```python
from build123d import *

# Parameters (mm, degrees)
CROQUIS1_W                 = 42
CROQUIS1_H                 = 68
CROQUIS1_W_2               = 34
CROQUIS1_H_2               = 60
SALIENTE_EXTRUIR1_DEPTH    = 60
CROQUIS2_R                 = 1.5
CORTAR_EXTRUIR1_DEPTH      = 39
CORTAR_EXTRUIR1_DEPTH_BACK = 5
CROQUIS3_W                 = 42
CROQUIS3_H                 = 68
SALIENTE_EXTRUIR2_DEPTH    = 4
CROQUIS4_W                 = 64
CROQUIS4_H                 = 20
SALIENTE_EXTRUIR3_DEPTH    = 42
SALIENTE_EXTRUIR4_DEPTH    = 64
SALIENTE_EXTRUIR6_DEPTH    = 64
CROQUIS8_R                 = 50
SALIENTE_EXTRUIR7_DEPTH    = 350
SALIENTE_EXTRUIR8_START    = -4
SALIENTE_EXTRUIR8_DEPTH    = 64
CROQUIS11_R                = 1.5
CORTAR_EXTRUIR2_DEPTH      = 68
CORTAR_EXTRUIR2_DEPTH_BACK = 34
CROQUIS13_R                = 10
CROQUIS13_R_2              = 50
SALIENTE_EXTRUIR9_DEPTH    = 20


with BuildPart() as part:
    # Croquis1 → Saliente-Extruir1 (new body)
    with BuildSketch(Plane.XY):
        Rectangle(CROQUIS1_W, CROQUIS1_H)
        Rectangle(CROQUIS1_W_2, CROQUIS1_H_2, mode=Mode.SUBTRACT)
    extrude(amount=SALIENTE_EXTRUIR1_DEPTH)

    # Croquis2 → Cortar-Extruir1 (cut, two sides)
    with BuildSketch(Plane(origin=(-17, 0, 0), x_dir=(0, 0, -1), z_dir=(1, 0, 0))) as cortar_extruir1_sk:
        with Locations((-49.779, -10)):
            Circle(CROQUIS2_R)
        with Locations((-46.914797213, -3.085202787)):
            Circle(CROQUIS2_R)
        with Locations((-40, -0.221)):
            Circle(CROQUIS2_R)
        with Locations((-33.085202787, -3.085202787)):
            Circle(CROQUIS2_R)
        with Locations((-30.221, -10)):
            Circle(CROQUIS2_R)
        with Locations((-33.085202787, -16.914797213)):
            Circle(CROQUIS2_R)
        with Locations((-40, -19.779)):
            Circle(CROQUIS2_R)
        with Locations((-46.914797213, -16.914797213)):
            Circle(CROQUIS2_R)
    extrude(amount=CORTAR_EXTRUIR1_DEPTH, mode=Mode.SUBTRACT)
    extrude(cortar_extruir1_sk.sketch, amount=-CORTAR_EXTRUIR1_DEPTH_BACK, mode=Mode.SUBTRACT)

    # Croquis3 → Saliente-Extruir2 (add)
    with BuildSketch(Plane(origin=(0, 0, 0), x_dir=(-1, 0, 0), z_dir=(0, 0, -1))):
        Rectangle(CROQUIS3_W, CROQUIS3_H)
    extrude(amount=SALIENTE_EXTRUIR2_DEPTH)

    # Croquis4 → Saliente-Extruir3 (add)
    with BuildSketch(Plane(origin=(21, 0, 0), x_dir=(0, 0, -1), z_dir=(1, 0, 0))):
        with Locations((-28, -44)):
            Rectangle(CROQUIS4_W, CROQUIS4_H)
    extrude(amount=-SALIENTE_EXTRUIR3_DEPTH)

    # Croquis5 → Saliente-Extruir4 (add)
    with BuildSketch(Plane(origin=(0, 0, -4), x_dir=(-1, 0, 0), z_dir=(0, 0, -1))):
        with BuildLine():
            ThreePointArc((21, 34), (0, 38.754486973), (-21, 34))
            Line((-21, 34), (21, 34))
        make_face()
        with BuildLine():
            ThreePointArc((-21, -54), (0, -58.754486973), (21, -54))
            Line((21, -54), (-21, -54))
        make_face()
    extrude(amount=-SALIENTE_EXTRUIR4_DEPTH)

    # Croquis6 → Saliente-Extruir6 (add)
    with BuildSketch(Plane(origin=(0, 0, -4), x_dir=(-1, 0, 0), z_dir=(0, 0, -1))):
        with BuildLine():
            Line((-21, 34), (21, 34))
            Line((21, 34), (21, 35.376205218))
            ThreePointArc((21, 35.376205218), (0, 40), (-21, 35.376205218))
            Line((-21, 35.376205218), (-21, 34))
        make_face()
        with BuildLine():
            Line((-21, -55.376205218), (-21, -54))
            Line((-21, -54), (21, -54))
            Line((21, -54), (21, -55.376205218))
            ThreePointArc((21, -55.376205218), (0, -60), (-21, -55.376205218))
        make_face()
    extrude(amount=-SALIENTE_EXTRUIR6_DEPTH)

    # Croquis8 → Saliente-Extruir7 (add)
    with BuildSketch(Plane(origin=(0, 0, -4), x_dir=(-1, 0, 0), z_dir=(0, 0, -1))):
        with Locations((0, -10)):
            Circle(CROQUIS8_R)
    extrude(amount=SALIENTE_EXTRUIR7_DEPTH)

    # Croquis10 → Saliente-Extruir8 (add)
    with BuildSketch(Plane.XY.offset(SALIENTE_EXTRUIR8_START)):
        with BuildLine():
            Line((-21, 35.376205218), (-21, -55.376205218))
            ThreePointArc((-21, -55.376205218), (-24.056410521, -53.832512053), (-27, -52.083250825))
            Line((-27, -52.083250825), (-27, 32.083250825))
            ThreePointArc((-27, 32.083250825), (-24.056410521, 33.832512053), (-21, 35.376205218))
        make_face()
        with BuildLine():
            Line((21, 35.376205218), (21, -55.376205218))
            ThreePointArc((21, -55.376205218), (24.056410521, -53.832512053), (27, -52.083250825))
            Line((27, -52.083250825), (27, 32.083250825))
            ThreePointArc((27, 32.083250825), (24.056410521, 33.832512053), (21, 35.376205218))
        make_face()
    extrude(amount=SALIENTE_EXTRUIR8_DEPTH)

    # Croquis11 → Cortar-Extruir2 (cut, two sides)
    with BuildSketch(Plane(origin=(-17, 0, 0), x_dir=(0, 0, -1), z_dir=(1, 0, 0))) as cortar_extruir2_sk:
        with Locations((-49.779, -10)):
            Circle(CROQUIS11_R)
        with Locations((-46.914797213, -3.085202787)):
            Circle(CROQUIS11_R)
        with Locations((-40, -0.221)):
            Circle(CROQUIS11_R)
        with Locations((-33.085202787, -3.085202787)):
            Circle(CROQUIS11_R)
        with Locations((-30.221, -10)):
            Circle(CROQUIS11_R)
        with Locations((-33.085202787, -16.914797213)):
            Circle(CROQUIS11_R)
        with Locations((-40, -19.779)):
            Circle(CROQUIS11_R)
        with Locations((-46.914797213, -16.914797213)):
            Circle(CROQUIS11_R)
    extrude(amount=CORTAR_EXTRUIR2_DEPTH, mode=Mode.SUBTRACT)
    extrude(cortar_extruir2_sk.sketch, amount=-CORTAR_EXTRUIR2_DEPTH_BACK, mode=Mode.SUBTRACT)

    # Croquis13 → Saliente-Extruir9 (add)
    with BuildSketch(Plane(origin=(0, 0, -354), x_dir=(-1, 0, 0), z_dir=(0, 0, -1))):
        with BuildLine():
            Line((-50, -80), (50, -80))
            ThreePointArc((50, -80), (64.142135624, -74.142135624), (70, -60))
            Line((70, -60), (70, 40))
            ThreePointArc((70, 40), (64.142135624, 54.142135624), (50, 60))
            Line((50, 60), (-50, 60))
            ThreePointArc((-50, 60), (-64.142135624, 54.142135624), (-70, 40))
            Line((-70, 40), (-70, -60))
            ThreePointArc((-70, -60), (-64.142135624, -74.142135624), (-50, -80))
        make_face()
        with Locations((-50, 40)):
            Circle(CROQUIS13_R, mode=Mode.SUBTRACT)
        with Locations((-50, -60)):
            Circle(CROQUIS13_R, mode=Mode.SUBTRACT)
        with Locations((50, 40)):
            Circle(CROQUIS13_R, mode=Mode.SUBTRACT)
        with Locations((50, -60)):
            Circle(CROQUIS13_R, mode=Mode.SUBTRACT)
        with Locations((0, -10)):
            Circle(CROQUIS13_R_2, mode=Mode.SUBTRACT)
    extrude(amount=-SALIENTE_EXTRUIR9_DEPTH)


solid = part.part
```
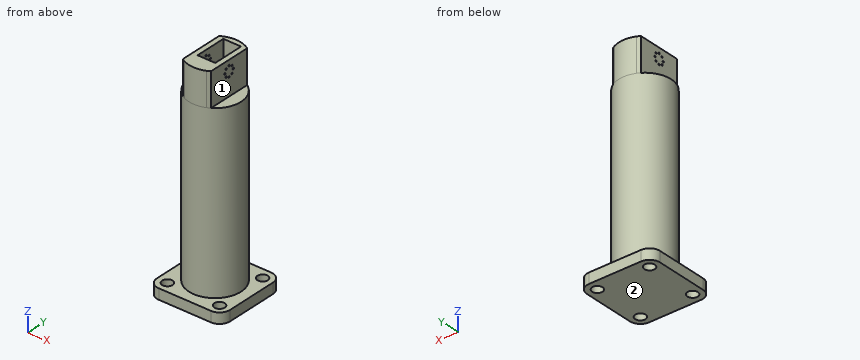
Build history of the part. All positions in model axes, mm. Face numbers are marked on the shaded views. A direction names the side the tool comes from. Coordinates: 2 decimals unless noted, no trailing zeros. Order: outer loops, then holes, each group sorted by start corner. A loop starts at its lowest first (then second) coordinate and runs counter-clockwise, first axis right, second up.
Item 1: Saw through at D-D on y = -44.5. List the corners of the cut face in (x, z), then the cut area to 3 significant figures.
Filled in:
outline: (-70, -354) - (70, -354) - (70, -334) - (36.19, -334) - (36.19, -4) - (27, -4) - (27, 60) - (-27, 60) - (-27, -4) - (-36.19, -4) - (-36.19, -334) - (-70, -334) - close
area: 30,100 mm2
Item 2: Saw through at B-B on z = -216.5. List the corners of the cut face in (x, y).
Filled in:
outline: circle Ø100 at (0, -10)
Item 3: Drop flat-ended pins along their axis: pin 1 Ø1 at (y, z) = (-4.5, -191.5) entering from +X; pin 2 Ø2 at (x, z) = (15, -85.5) entering from -Y; pin 3 Ø4 at (y, z) = (-10, 49.779) entering from +X. Give the stop position or say it passes through.
Filled in:
pin 1: stops at x = 49.75
pin 2: stops at y = -58
pin 3: stops at x = 27
Item 4: Saw through at A-A on y = 20. List the corners of the cut face in (x, z).
Filled in:
outline: (-70, -354) - (70, -354) - (70, -334) - (40, -334) - (40, -4) - (27, -4) - (27, 60) - (17, 60) - (17, 0) - (-17, 0) - (-17, 60) - (-27, 60) - (-27, -4) - (-40, -4) - (-40, -334) - (-70, -334) - close
Item 5: Tool access for the marked faces 1 and 2: list every direction of +Z, -Z, +X, -X, +Y, -Y with a clear straight run to the whole face (end or side of a thin tool).
Filled in:
face 1: +Z, +X, +Y, -Y
face 2: -Z, +X, -X, +Y, -Y
Item 6: Drill centre lines: L1, parallel to Z at x = 23.75, y = -10; L2, parallel to X at y = 17, z = 35; L3, parallel to Y at x = 50, z = -345.25. Where is each one in solid material? Low to high.
Filled in:
L1: z = -354 to 28.72, 31.72 to 48.28, 51.28 to 60
L2: x = -27 to -17, 17 to 27
L3: y = -80 to -70, -50 to 30, 50 to 60
Item 7: Saw through at C-C on x = -35. List the corners of the cut face in (y, z), then the cut area to 3 significant figures.
Filled in:
outline: (-80, -354) - (60, -354) - (60, -334) - (25.71, -334) - (25.71, -4) - (-45.71, -4) - (-45.71, -334) - (-80, -334) - close
area: 26,400 mm2
